from build123d import *

# Parameters (mm, degrees)
SKETCH3_W         = 0.8128
SKETCH3_H         = 3.6322
SKETCH4_W         = 0.4064
SKETCH4_H         = 0.4064
CIRPATTERN1_COUNT = 2
CIRPATTERN1_ANGLE = 90
CHAMFER1_SIZE     = 0.254


with BuildPart() as part:
    # BodySke → Base-Revolve (revolve)
    with BuildSketch(Plane.XY, mode=Mode.PRIVATE) as base_revolve_sk:
        with BuildLine():
            Line((2.032, 1.4224), (2.032, 2.7813))
            Line((2.032, 2.7813), (1.075646615, 2.7813))
            ThreePointArc((1.075646615, 2.7813), (0.960371669, 2.753635341), (0.87020729, 2.676667612))
            ThreePointArc((0.87020729, 2.676667612), (0.223015279, 1.407285528), (0, 0))
            Line((0, 0), (21.082, 0))
            Line((21.082, 0), (21.082, 1.4224))
            Line((21.082, 1.4224), (2.032, 1.4224))
        make_face()
    revolve(base_revolve_sk.sketch.rotate(Axis((-25.4, 0, 0), (1, 0, 0)), 90), axis=Axis((-25.4, 0, 0), (1, 0, 0)))  # turned: the seam where the file's is

    # Sketch3 → Cut-Loft1 section 0
    with BuildSketch(Plane(origin=(0, 0, 0), x_dir=(0, 0, -1), z_dir=(1, 0, 0))):
        Rectangle(SKETCH3_W, SKETCH3_H)
    # Sketch4 → Cut-Loft1 section 1
    with BuildSketch(Plane(origin=(2.0066, 0, 0), x_dir=(0, 0, -1), z_dir=(1, 0, 0))):
        Rectangle(SKETCH4_W, SKETCH4_H)
    cut_loft1 = loft(mode=Mode.SUBTRACT)

    # CirPattern1: Cut-Loft1 ×2 about axis
    cirpattern1_axis = Axis((0, 0, 0), (1, 0, 0))
    for i in range(1, CIRPATTERN1_COUNT):
        add(cut_loft1.rotate(cirpattern1_axis, i * CIRPATTERN1_ANGLE / (CIRPATTERN1_COUNT - 1)), mode=Mode.SUBTRACT)

    # Chamfer1
    chamfer1_edges = [part.edges().sort_by_distance(p)[0] for p in [
        (21.082, 0, -1.4224),
    ]]
    chamfer(chamfer1_edges, length=CHAMFER1_SIZE)


solid = part.part
Could you check a few things on this model? Use its own coordinates, in mm. A direction names the side the tool comes from. Coordinates: 2 decimals unless noted, no trailing zeros. Order: outer loops, then holes, each group sorted by start corner. A loop starts at its lowest first (then second) coordinate and runs counter-clockwise, first axis right, second up.
Q1. Which directions (+Z, -Z, +X, -X, +Y, -Y) give clear straight access to the entire face, cutting with the end or side of a thin tool? Please do faces 1 (the flat face through (21.082, 0, 0)), 2 (the cylindrical face through (11.3, 1.26, 0.66)).
Q2. Please list where these lines run through material, in increasing order: L1, parallel to X at y = -1.8, z = 0.8; L2, parallel to X at y = 0.5, z = 0.15; L3, parallel to Z at x = 3.25, y = -1.05.
Q3. Will these pins go through, and if not, where does the flat tip stop? pin 1 (1 mm diameter, centred on x = 6.5, y = -0.5, fed in from -Z); pin 2 (1.5 mm diameter, centred on x = 15, y = 1.5, fed in from +Z); pin 3 (1.5 mm diameter, centred on y = 1.5, z = 1.5, fed in from +X).
Q4. Suppose I cut it at A-A on x = 10.5. Please give me the cut outline in (y, z), and give its area (3 significant figures).
Answer:
1. face 1: +Z, -Z, +X, +Y, -Y
1. face 2: +X
2. L1: x = 0.45 to 2.03
2. L2: x = 1.64 to 21.08
2. L3: z = -0.96 to 0.96
3. pin 1: stops at z = -1.42
3. pin 2: stops at z = 1.21
3. pin 3: stops at x = 20.88
4. outline: circle Ø2.84 at (0, 0)
4. area: 6.36 mm2
